Geometry: final body of the model. Coordinates: model frame, mm. Give positions to 0.01 mm unless a question says otherwise; leave off trailing zeros. One line per question, with ' | ' between items.
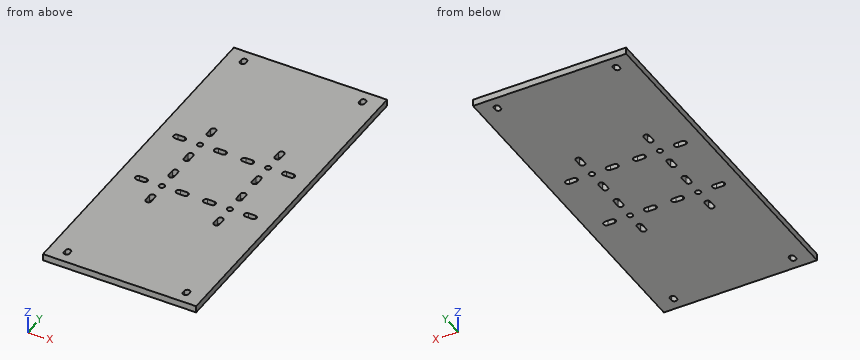
from build123d import *

# Parameters (mm, degrees)
SKETCH_1_W      = 180
SKETCH_1_H      = 384
SKETCH_1_R      = 3.25
EXTRUDE_1_DEPTH = 8
SKETCH_2_W      = 180
SKETCH_2_H      = 8
EXTRUDE_2_DEPTH = 8
SKETCH_3_W      = 180
SKETCH_3_H      = 8
EXTRUDE_3_DEPTH = 8


with BuildPart() as part:
    # 草图1 → 凸台-拉伸1 (new body)
    with BuildSketch(Plane.XY):
        with Locations((0, 177)):
            Rectangle(SKETCH_1_W, SKETCH_1_H)
        with Locations((40, 217)):
            Circle(SKETCH_1_R, mode=Mode.SUBTRACT)
        with Locations(Location((-40, 217, 0), (0, 0, 180))):
            Circle(SKETCH_1_R, mode=Mode.SUBTRACT)
        with Locations(Location((40, 137, 0), (0, 0, 180))):
            Circle(SKETCH_1_R, mode=Mode.SUBTRACT)
        with Locations((-40, 137)):
            Circle(SKETCH_1_R, mode=Mode.SUBTRACT)
        with BuildLine():
            Line((-73.25, 360), (-73.25, 363))
            ThreePointArc((-73.25, 363), (-70, 366.25), (-66.75, 363))
            Line((-66.75, 363), (-66.75, 360))
            ThreePointArc((-66.75, 360), (-70, 356.75), (-73.25, 360))
        make_face(mode=Mode.SUBTRACT)
        with BuildLine():
            Line((73.25, 360), (73.25, 363))
            ThreePointArc((73.25, 363), (70, 366.25), (66.75, 363))
            Line((66.75, 363), (66.75, 360))
            ThreePointArc((66.75, 360), (70, 356.75), (73.25, 360))
        make_face(mode=Mode.SUBTRACT)
        with BuildLine():
            Line((-73.25, -6), (-73.25, -9))
            ThreePointArc((-73.25, -9), (-70, -12.25), (-66.75, -9))
            Line((-66.75, -9), (-66.75, -6))
            ThreePointArc((-66.75, -6), (-70, -2.75), (-73.25, -6))
        make_face(mode=Mode.SUBTRACT)
        with BuildLine():
            Line((73.25, -6), (73.25, -9))
            ThreePointArc((73.25, -9), (70, -12.25), (66.75, -9))
            Line((66.75, -9), (66.75, -6))
            ThreePointArc((66.75, -6), (70, -2.75), (73.25, -6))
        make_face(mode=Mode.SUBTRACT)
        with BuildLine():
            Line((12, 220.25), (20, 220.25))
            ThreePointArc((20, 220.25), (23.25, 217), (20, 213.75))
            Line((20, 213.75), (12, 213.75))
            ThreePointArc((12, 213.75), (8.75, 217), (12, 220.25))
        make_face(mode=Mode.SUBTRACT)
        with BuildLine():
            Line((43.25, 245), (43.25, 237))
            ThreePointArc((43.25, 237), (40, 233.75), (36.75, 237))
            Line((36.75, 237), (36.75, 245))
            ThreePointArc((36.75, 245), (40, 248.25), (43.25, 245))
        make_face(mode=Mode.SUBTRACT)
        with BuildLine():
            Line((-43.25, 245), (-43.25, 237))
            ThreePointArc((-43.25, 237), (-40, 233.75), (-36.75, 237))
            Line((-36.75, 237), (-36.75, 245))
            ThreePointArc((-36.75, 245), (-40, 248.25), (-43.25, 245))
        make_face(mode=Mode.SUBTRACT)
        with BuildLine():
            Line((-12, 220.25), (-20, 220.25))
            ThreePointArc((-20, 220.25), (-23.25, 217), (-20, 213.75))
            Line((-20, 213.75), (-12, 213.75))
            ThreePointArc((-12, 213.75), (-8.75, 217), (-12, 220.25))
        make_face(mode=Mode.SUBTRACT)
        with BuildLine():
            Line((-36.75, 189), (-36.75, 197))
            ThreePointArc((-36.75, 197), (-40, 200.25), (-43.25, 197))
            Line((-43.25, 197), (-43.25, 189))
            ThreePointArc((-43.25, 189), (-40, 185.75), (-36.75, 189))
        make_face(mode=Mode.SUBTRACT)
        with BuildLine():
            Line((-68, 213.75), (-60, 213.75))
            ThreePointArc((-60, 213.75), (-56.75, 217), (-60, 220.25))
            Line((-60, 220.25), (-68, 220.25))
            ThreePointArc((-68, 220.25), (-71.25, 217), (-68, 213.75))
        make_face(mode=Mode.SUBTRACT)
        with BuildLine():
            Line((68, 213.75), (60, 213.75))
            ThreePointArc((60, 213.75), (56.75, 217), (60, 220.25))
            Line((60, 220.25), (68, 220.25))
            ThreePointArc((68, 220.25), (71.25, 217), (68, 213.75))
        make_face(mode=Mode.SUBTRACT)
        with BuildLine():
            Line((36.75, 189), (36.75, 197))
            ThreePointArc((36.75, 197), (40, 200.25), (43.25, 197))
            Line((43.25, 197), (43.25, 189))
            ThreePointArc((43.25, 189), (40, 185.75), (36.75, 189))
        make_face(mode=Mode.SUBTRACT)
        with BuildLine():
            Line((-68, 140.25), (-60, 140.25))
            ThreePointArc((-60, 140.25), (-56.75, 137), (-60, 133.75))
            Line((-60, 133.75), (-68, 133.75))
            ThreePointArc((-68, 133.75), (-71.25, 137), (-68, 140.25))
        make_face(mode=Mode.SUBTRACT)
        with BuildLine():
            Line((-43.25, 109), (-43.25, 117))
            ThreePointArc((-43.25, 117), (-40, 120.25), (-36.75, 117))
            Line((-36.75, 117), (-36.75, 109))
            ThreePointArc((-36.75, 109), (-40, 105.75), (-43.25, 109))
        make_face(mode=Mode.SUBTRACT)
        with BuildLine():
            Line((-12, 133.75), (-20, 133.75))
            ThreePointArc((-20, 133.75), (-23.25, 137), (-20, 140.25))
            Line((-20, 140.25), (-12, 140.25))
            ThreePointArc((-12, 140.25), (-8.75, 137), (-12, 133.75))
        make_face(mode=Mode.SUBTRACT)
        with BuildLine():
            Line((-36.75, 165), (-36.75, 157))
            ThreePointArc((-36.75, 157), (-40, 153.75), (-43.25, 157))
            Line((-43.25, 157), (-43.25, 165))
            ThreePointArc((-43.25, 165), (-40, 168.25), (-36.75, 165))
        make_face(mode=Mode.SUBTRACT)
        with BuildLine():
            Line((43.25, 109), (43.25, 117))
            ThreePointArc((43.25, 117), (40, 120.25), (36.75, 117))
            Line((36.75, 117), (36.75, 109))
            ThreePointArc((36.75, 109), (40, 105.75), (43.25, 109))
        make_face(mode=Mode.SUBTRACT)
        with BuildLine():
            Line((12, 133.75), (20, 133.75))
            ThreePointArc((20, 133.75), (23.25, 137), (20, 140.25))
            Line((20, 140.25), (12, 140.25))
            ThreePointArc((12, 140.25), (8.75, 137), (12, 133.75))
        make_face(mode=Mode.SUBTRACT)
        with BuildLine():
            Line((68, 140.25), (60, 140.25))
            ThreePointArc((60, 140.25), (56.75, 137), (60, 133.75))
            Line((60, 133.75), (68, 133.75))
            ThreePointArc((68, 133.75), (71.25, 137), (68, 140.25))
        make_face(mode=Mode.SUBTRACT)
        with BuildLine():
            Line((36.75, 165), (36.75, 157))
            ThreePointArc((36.75, 157), (40, 153.75), (43.25, 157))
            Line((43.25, 157), (43.25, 165))
            ThreePointArc((43.25, 165), (40, 168.25), (36.75, 165))
        make_face(mode=Mode.SUBTRACT)
    extrude(amount=EXTRUDE_1_DEPTH)

    # 草图2 → 凸台-拉伸2 (add)
    with BuildSketch(Plane(origin=(0, 369, 0), x_dir=(1, 0, 0), z_dir=(0, 1, 0))):
        with Locations((0, -4)):
            Rectangle(SKETCH_2_W, SKETCH_2_H)
    extrude(amount=EXTRUDE_2_DEPTH)

    # 草图3 → 凸台-拉伸3 (add)
    with BuildSketch(Plane.XZ.offset(15)):
        with Locations((0, 4)):
            Rectangle(SKETCH_3_W, SKETCH_3_H)
    extrude(amount=EXTRUDE_3_DEPTH)


solid = part.part
1) Contact query for a flat-ended pin moving along its axis: pin 1 Ø12 at (x, y) = (56, 184.5) entering from -Z. Output: stop coordinate, or through.
Check result:
pin 1: stops at z = 0
2) Material intervals for probe 1 along Y at (x, z) = (-62, 4.75); probe 2 along X at (y, z) = (197, 1), sorted ascending. Write a range as from..to.
Check result:
probe 1: y = -23..133.75, 140.25..213.75, 220.25..377 | probe 2: x = -90..-43.25, -36.75..36.75, 43.25..90
3) Section A-A on z = 5.5. Count the separate pieces of the cut face and the enclosed holes in it, plus the area to 3 significant figures.
Check result:
separate pieces: 1 | enclosed holes: 24 | area: 70,300 mm^2
